Here's how the part is built. I have some questions about the finished solid (model axes, mm). A direction names the side the tool comes from. Give positions to 0.01 mm unless a question says otherwise; leave off trailing zeros. Loops run counter-clockwise (first coordinate to the right, second up) from the corner with the lowest first, then second, coordinate; pieces in that order, holes last. Notation, with made-up numbers: (89.25, 37.25) - (97.25, 37.25) arc R33 cw to (97.25, 73.25) - close; hole circle Ø7 at (21.5, 61.5). An arc over 180 degrees is marked (long way). One line per item, written item: value. Start each with the question number.
Autodesk Inventor part; units mm, degrees
ref_plane "rot_XY" through (0, 6.6675, 0) normal (0, 0, 1) x (1, 0, 0)
ref_plane "rot_YZ" through (0, 6.6675, 0) normal (1, 0, 0) x (0, 1, 0)
ref_plane "rot_ZX" through (0, 6.6675, 0) normal (0, 1, 0) x (0, 0, 1)
sketch "Sketch_2" plane through (0, -0.254, 0) normal (0, 1, 0) x (1, 0, 0)
  line L0 (-6.5024, -6.35) -> (-6.0389, -6.35)
  line L1 (-6.0389, -6.35) -> (-6.0389, -5.8865)
  line L2 (-6.0389, -5.8865) -> (-3.2509, -5.8865)
  line L3 (-3.2509, -5.8865) -> (-3.0348, -5.4229)
  line L4 (-3.0348, -5.4229) -> (-2.0452, -5.4229)
  line L5 (-2.0452, -5.4229) -> (-1.8291, -5.8865)
  line L6 (-1.8291, -5.8865) -> (1.8291, -5.8865)
  line L7 (1.8291, -5.8865) -> (2.0452, -5.4229)
  line L8 (2.0452, -5.4229) -> (3.0348, -5.4229)
  line L9 (3.0348, -5.4229) -> (3.2509, -5.8865)
  line L10 (3.2509, -5.8865) -> (6.0389, -5.8865)
  line L11 (6.0389, -5.8865) -> (6.0389, -6.35)
  line L12 (6.0389, -6.35) -> (6.5024, -6.35)
  line L13 (6.5024, -6.35) -> (6.5024, 6.35)
  line L14 (6.5024, 6.35) -> (6.0389, 6.35)
  line L15 (6.0389, 6.35) -> (6.0389, 5.8865)
  line L16 (6.0389, 5.8865) -> (3.2509, 5.8865)
  line L17 (3.2509, 5.8865) -> (3.0348, 5.4229)
  line L18 (3.0348, 5.4229) -> (2.0452, 5.4229)
  line L19 (2.0452, 5.4229) -> (1.8291, 5.8865)
  line L20 (1.8291, 5.8865) -> (-1.8291, 5.8865)
  line L21 (-1.8291, 5.8865) -> (-2.0452, 5.4229)
  line L22 (-2.0452, 5.4229) -> (-3.0348, 5.4229)
  line L23 (-3.0348, 5.4229) -> (-3.2509, 5.8865)
  line L24 (-3.2509, 5.8865) -> (-6.0389, 5.8865)
  line L25 (-6.0389, 5.8865) -> (-6.0389, 6.35)
  line L26 (-6.0389, 6.35) -> (-6.5024, 6.35)
  line L27 (-6.5024, 6.35) -> (-6.5024, -6.35)
extrude "Extrusion1" add sketch "Sketch_2" against normal blind 9.8476
sketch "Sketch_8" plane through (0, -9.5936, 0) normal (0, 1, 0) x (1, 0, 0)
  line L0 (-5.08, -2.794) -> (-4.318, -2.794)
  line L1 (-4.318, -2.794) -> (-4.318, -1.016)
  line L2 (-4.318, -1.016) -> (-5.08, -1.016)
  line L3 (-5.08, -1.016) -> (-5.08, -2.794)
extrude "Extrusion2" cut sketch "Sketch_8" against normal blind 25.4
sketch "Sketch_5" plane through (0, -9.5936, 0) normal (0, 1, 0) x (1, 0, 0)
  line L0 (-0.381, -2.794) -> (0.381, -2.794)
  line L1 (0.381, -2.794) -> (0.381, -1.016)
  line L2 (0.381, -1.016) -> (-0.381, -1.016)
  line L3 (-0.381, -1.016) -> (-0.381, -2.794)
extrude "Extrusion3" cut sketch "Sketch_5" against normal blind 25.4
sketch "Sketch_9" plane through (0, -9.5936, 0) normal (0, 1, 0) x (1, 0, 0)
  line L0 (4.318, -2.794) -> (5.08, -2.794)
  line L1 (5.08, -2.794) -> (5.08, -1.016)
  line L2 (5.08, -1.016) -> (4.318, -1.016)
  line L3 (4.318, -1.016) -> (4.318, -2.794)
extrude "Extrusion4" cut sketch "Sketch_9" against normal blind 25.4
sketch "Sketch_10" plane through (0, -9.5936, 0) normal (0, 1, 0) x (1, 0, 0)
  line L0 (-5.08, 1.016) -> (-4.318, 1.016)
  line L1 (-4.318, 1.016) -> (-4.318, 2.794)
  line L2 (-4.318, 2.794) -> (-5.08, 2.794)
  line L3 (-5.08, 2.794) -> (-5.08, 1.016)
extrude "Extrusion5" cut sketch "Sketch_10" against normal blind 25.4
sketch "Sketch_11" plane through (0, -9.5936, 0) normal (0, 1, 0) x (1, 0, 0)
  line L0 (-0.381, 1.016) -> (0.381, 1.016)
  line L1 (0.381, 1.016) -> (0.381, 2.794)
  line L2 (0.381, 2.794) -> (-0.381, 2.794)
  line L3 (-0.381, 2.794) -> (-0.381, 1.016)
extrude "Extrusion6" cut sketch "Sketch_11" against normal blind 25.4
sketch "Sketch_12" plane through (0, -9.5936, 0) normal (0, 1, 0) x (1, 0, 0)
  line L0 (4.318, 1.016) -> (5.08, 1.016)
  line L1 (5.08, 1.016) -> (5.08, 2.794)
  line L2 (5.08, 2.794) -> (4.318, 2.794)
  line L3 (4.318, 2.794) -> (4.318, 1.016)
extrude "Extrusion7" cut sketch "Sketch_12" against normal blind 25.4
sketch "Sketch_19" plane through (0, -0.254, 0) normal (0, 1, 0) x (1, 0, 0)
  line L0 (-6.5024, -6.35) -> (-6.0389, -6.35)
  line L1 (-6.0389, -6.35) -> (-6.0389, -5.8865)
  line L2 (-6.0389, -5.8865) -> (-3.2509, -5.8865)
  line L3 (-3.2509, -5.8865) -> (-3.0348, -5.4229)
  line L4 (-3.0348, -5.4229) -> (-2.0452, -5.4229)
  line L5 (-2.0452, -5.4229) -> (-1.8291, -5.8865)
  line L6 (-1.8291, -5.8865) -> (1.8291, -5.8865)
  line L7 (1.8291, -5.8865) -> (2.0452, -5.4229)
  line L8 (2.0452, -5.4229) -> (3.0348, -5.4229)
  line L9 (3.0348, -5.4229) -> (3.2509, -5.8865)
  line L10 (3.2509, -5.8865) -> (6.0389, -5.8865)
  line L11 (6.0389, -5.8865) -> (6.0389, -6.35)
  line L12 (6.0389, -6.35) -> (6.5024, -6.35)
  line L13 (6.5024, -6.35) -> (6.5024, 6.35)
  line L14 (6.5024, 6.35) -> (6.0389, 6.35)
  line L15 (6.0389, 6.35) -> (6.0389, 5.8865)
  line L16 (6.0389, 5.8865) -> (3.2509, 5.8865)
  line L17 (3.2509, 5.8865) -> (3.0348, 5.4229)
  line L18 (3.0348, 5.4229) -> (2.0452, 5.4229)
  line L19 (2.0452, 5.4229) -> (1.8291, 5.8865)
  line L20 (1.8291, 5.8865) -> (-1.8291, 5.8865)
  line L21 (-1.8291, 5.8865) -> (-2.0452, 5.4229)
  line L22 (-2.0452, 5.4229) -> (-3.0348, 5.4229)
  line L23 (-3.0348, 5.4229) -> (-3.2509, 5.8865)
  line L24 (-3.2509, 5.8865) -> (-6.0389, 5.8865)
  line L25 (-6.0389, 5.8865) -> (-6.0389, 6.35)
  line L26 (-6.0389, 6.35) -> (-6.5024, 6.35)
  line L27 (-6.5024, 6.35) -> (-6.5024, -6.35)
extrude "Extrusion8" cut sketch "Sketch_19" against normal blind 0.254
ref_plane "rot_XY" through (0, 6.6675, 0) normal (0, 0, 1) x (1, 0, 0)
ref_plane "rot_YZ" through (0, 6.6675, 0) normal (1, 0, 0) x (0, 1, 0)
ref_plane "rot_ZX" through (0, 6.6675, 0) normal (0, 1, 0) x (0, 0, 1)
ref_plane "to_cover_XY" through (0, -0.254, 0) normal (0, 1, 0) x (1, 0, 0)
ref_plane "to_cover_YZ" through (0, -0.254, 0) normal (1, 0, 0) x (0, 0, -1)
ref_plane "to_cover_ZX" through (0, -0.254, 0) normal (0, 0, -1) x (0, 1, 0)
ref_plane "to_terminals_XY" through (0, -9.5936, 0) normal (0, -1, 0) x (1, 0, 0)
ref_plane "to_terminals_YZ" through (0, -9.5936, 0) normal (1, 0, 0) x (0, 0, 1)
ref_plane "to_terminals_ZX" through (0, -9.5936, 0) normal (0, 0, 1) x (0, -1, 0)
properties part number "M20_ang2830TX-switch"
(1) If we section it at B-B on x = -4.5: List the corners of the cut face in (y, z) for me.
(2) Please list where these lines run through material, in increasing order: probe 1 along X at (y, z) = (-6.75, -5.5); probe 2 along Z at (x, y) = (-5.25, -0.75); probe 3 along Z at (x, y) = (-3, -1.75). Write a range as from..to.
(3) Will these pins go through, and if not, where does the flat tip stop? pin 1 (0.8 mm diameter, centred on x = 2.5, y = -5.5, fed in from +Z); pin 2 (1.5 mm diameter, centred on x = -4.5, y = -5, fed in from +Z); pin 3 (0.6 mm diameter, centred on x = 5, z = -1.5, fed in from -Y); pin 4 (0.5 mm diameter, centred on x = 2.5, y = -5, fed in from -Z).
(4) For faces 4 (the face through (0, -10.102, 0)), 5 (the face through (0, -5, 5.886)), 6 (the face through (0, -5, -5.886)), which set-ups out of +Z, -Z, +X, -X, +Y, -Y let a thin tool reach every point of the face, with its end or its side?
(5) If we section it at A-A on y = -1.5: List the corners of the cut face in (x, z) for me.
(6) If we mould it in two halves opening along X, with no side actions, what happens to faces 1 (the face through (-6.502, -5, 0)), 2 (the face through (-5, -5, -5.886)), 3 (the face through (0, -0.508, 0))? For each: pulls with the +X half, pulls with the -X half, needs draft (parallel to the pull), parting line crosses it, or undercut.
(7) If we section it at C-C on x = -1.5: List the corners of the cut face in (y, z) for me, plus the area to 3 significant figures.
Found:
1. outline: (-10.1, -5.89) - (-0.51, -5.89) - (-0.51, 5.89) - (-10.1, 5.89) - (-10.1, 2.79) - (-9.59, 2.79) - (-9.59, 1.02) - (-10.1, 1.02) - (-10.1, -1.02) - (-9.59, -1.02) - (-9.59, -2.79) - (-10.1, -2.79) - close
2. probe 1: -6.5..-3.07, -2.01..2.01, 3.07..6.5
2. probe 2: -5.89..5.89
2. probe 3: -5.42..5.42
3. pin 1: z = 5.42
3. pin 2: z = 5.89
3. pin 3: y = -10.1
3. pin 4: z = -5.42
4. face 4: +Z, -Z, +X, -X, -Y
4. face 5: +Z, +Y, -Y
4. face 6: -Z, +Y, -Y
5. outline: (-6.5, -6.35) - (-6.04, -6.35) - (-6.04, -5.89) - (-3.25, -5.89) - (-3.03, -5.42) - (-2.05, -5.42) - (-1.83, -5.89) - (1.83, -5.89) - (2.05, -5.42) - (3.03, -5.42) - (3.25, -5.89) - (6.04, -5.89) - (6.04, -6.35) - (6.5, -6.35) - (6.5, 6.35) - (6.04, 6.35) - (6.04, 5.89) - (3.25, 5.89) - (3.03, 5.42) - (2.05, 5.42) - (1.83, 5.89) - (-1.83, 5.89) - (-2.05, 5.42) - (-3.03, 5.42) - (-3.25, 5.89) - (-6.04, 5.89) - (-6.04, 6.35) - (-6.5, 6.35) - close
6. face 1: pulls with the -X half
6. face 2: undercut
6. face 3: needs draft
7. outline: (-10.1, -5.89) - (-0.51, -5.89) - (-0.51, 5.89) - (-10.1, 5.89) - close
7. area: 113 mm^2
